The listing builds one solid part. Answer for the finished solid, in the listing's coordinates (mm). Round coordinates to 2 decimals unless told otherwise and drop trailing zeros. Write each loop counter-clockwise with the first axis right and the second up, starting at its lowest first coordinate (ties: lowest second). Pieces come first, ordered by that corner, then holes. Notation, with made-up numbers: M -19,-28 L 4,-28 A19 ccw 4,-1 Z; hole C 40,37 d4. An arc over 180 degrees is marked long. One line per item, written item: value. Start each with the question number.
(1) Section B-B (y = 37) is taken. Determine the outline of the cut face in (x, z).
(2) Consider probe 1 along Y at (x, z) = (0.25, 8); probe 2 along X at (y, z) = (0, 4.75); probe 3 along Y at (x, z) = (4.25, 6.5). Determine where each line is inside the solid, lowest interval first.
(3) Section C-C (x = -8) is taken. Determine the outline of the cut face in (y, z), plus the area to 3 significant figures.
(4) Given P1, Ø4.5, axis at y = 15.5, z = 4, coming from the +X side; P2, Ø1, axis at x = 6.5, z = 7, coming from the -Y side; P3, Ø4, axis at y = 64.5, z = 6, coming from the -X side; P4, Ø1, axis at y = -11, z = 1.5, coming from the +X side, each flat-ended and moving along its own axis, determine where each tip first touches the part or whether it passes through.
(5) Section A-A (y = 0) is taken. Determine the outline of the cut face in (x, z).
Autodesk Fusion 360 part; units mm, degrees
sketch "Szkic1" plane through (0, 0, 0) normal (0, 0, 1) x (1, 0, 0)
  circle A0 centre (0, 0) radius 5.5
  line L0 (-3, 150) -> (3, 150)
  line L1 (3, 150) -> (3, -30)
  line L2 (3, -30) -> (-3, -30)
  line L3 (-3, -30) -> (-3, 150)
  line L4 (0, 1.75) -> (0, 22.5)
  circle A1 centre (0, 0) radius 10
  dimension "d7" = 11
  dimension "d8" = 30
  dimension "d10" = 6
  dimension "d11" = 180
  dimension "d12" = 20
extrude "Wyciągnięcie proste1" add sketch "Szkic1" along normal blind 10 contours A0 L1 A1 | A0 L1 L4 A1 | A0 L1 L3 A1 | A0 L3 L4 A1 | A0 L3 A1
extrude "Wyciągnięcie proste2" add sketch "Szkic1" along normal blind 5 from surface at 2.5 contours L0 L1 L3 A1 | L1 L2 L3 A1
ref_plane "Płaszczyzna konstrukcyjna1" through (0, -19.7697, 5) normal (0, 0, 1) x (1, 0, 0)
sketch "Szkic2" plane through (0, 0, 5) normal (0, 0, 1) x (1, 0, 0)
  circle A0 centre (6, 25) radius 2.5
  line L0 (4.9, 22.755) -> (3, 22.755)
  line L1 (3, 22.755) -> (3, 27.245)
  line L2 (3, 27.245) -> (4.9, 27.245)
  line L3 (4.9, 27.245) -> (4.9, 22.755)
  line L4 (3, 150) -> (3, -30)
  line L5 (6, 25) -> (3, 25)
  line L6 (7.25, 22.8349) -> (7.25, 27.1651)
  circle A1 centre (6, 25) radius 1.75
  line L7 (7.7321, 24.75) -> (6, 24.75)
  line L8 (6, 24.75) -> (6, 25.25)
  line L9 (6, 25.25) -> (7.7321, 25.25)
  line L10 (7.7321, 25.25) -> (7.7321, 24.75)
  line L11 (-3, 150) -> (3, 150)
  dimension "d18" = 5
  dimension "d19" = 1.25
  dimension "d20" = 3.5
  dimension "d21" = 0.5
  dimension "d22" = 25
  dimension "d23" = 125
  dimension "d24" = 1.1
  dimension "d25" = 3
revolve "Obrót1" add sketch "Szkic2" angle 360 about axis through (6, 25, 5) along (-1, 0, 0) contours A0 L3 L6 A1 | A0 L0 L1 L4 L5 | A0 L3 L5 A1 picked at (5.1557, 22.9188) picked at (4.6078, 23.2377)
extrude "Wyciągnięcie proste3" cut sketch "Szkic2" along normal through all and the other way through all contours L6 L7 L8 L9
pattern_circular "Szyk kołowy1" count 2 over 90 about axis through (6, 25, 5) along (-1, 0, 0) of "Wyciągnięcie proste3"
fillet "Zaokrąglenie1" radius 0.5 15 edges at (3, 79.7697, 7.5) (-3, 79.7697, 7.5) (3, 79.7697, 2.5) (-3, 79.7697, 2.5) (3, -19.7697, 7.5) (-3, -19.7697, 7.5) (3, -19.7697, 2.5) (-3, -19.7697, 2.5) (-3, -30, 5) (0, -30, 7.5) (3, -30, 5) (0, -30, 2.5) (0, 150, 7.5) (-3, 150, 5) (0, 150, 2.5)
fillet "Zaokrąglenie1" radius 4 1 edges at (3, 150, 5)
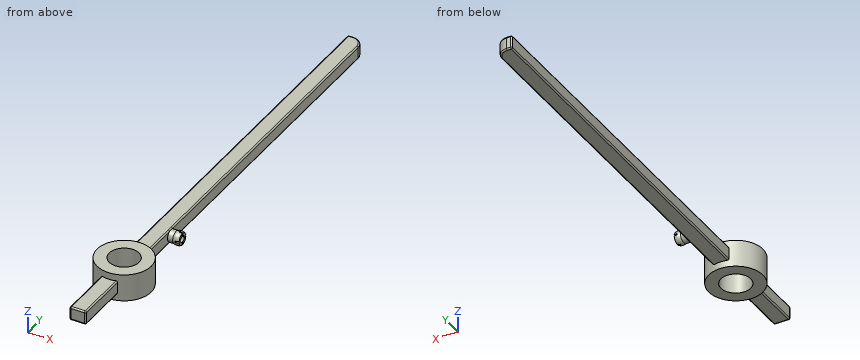
Recorded:
1. outline: M -3,3 A0.5 ccw -2.5,2.5 L 2.5,2.5 A0.5 ccw 3,3 L 3,7 A0.5 ccw 2.5,7.5 L -2.5,7.5 A0.5 ccw -3,7 Z
2. probe 1: y = -10 to -5.49, 5.49 to 10
2. probe 2: x = -10 to -5.5, 5.5 to 10
2. probe 3: y = -9.05 to -3.49, 3.49 to 9.05, 23.33 to 26.67
3. outline: M -6,0 L 6,0 L 6,10 L -6,10 Z
3. area: 120 mm2
4. P1: stops at x = 3
4. P2: stops at y = -8
4. P3: stops at x = -3
4. P4: passes through
5. outline: M -10,0 L -5.5,0 L -5.5,10 L -10,10 Z; M 5.5,0 L 10,0 L 10,10 L 5.5,10 Z
